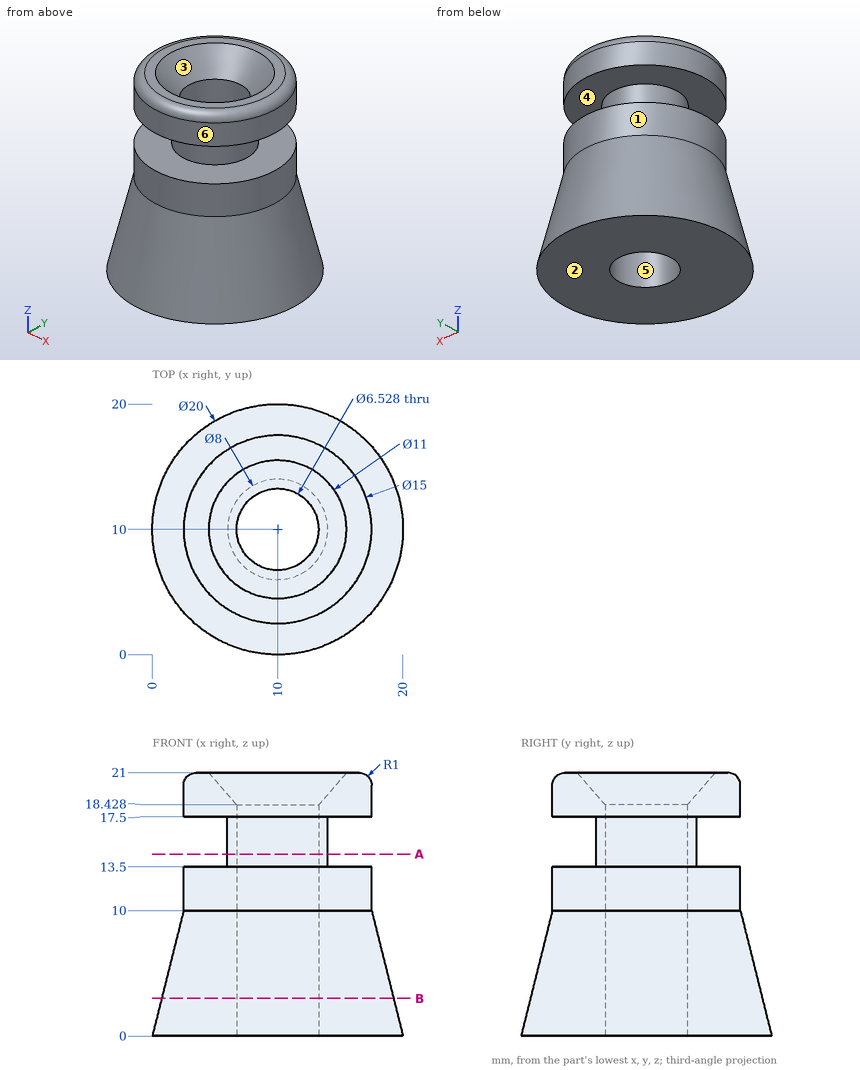
The drawing under review shows one solid part. Ordinate dimensions are in mm from its lowest x, y, z. A direction names the side the tool comes from. Round coordinates to 2 decimals unless told otherwise and drop trailing zeros. Write each loop counter-clockwise with the first axis right and the second up, starting at its lowest first coordinate (ties: lowest second). Pieces come first, ordered by that corner, then holes. Notation, with made-up numbers: (22.5, 60.5) -> (71.5, 60.5) arc R12 ccw to (71.5, 64.5) -> close; hole circle Ø4 at (-23, 38). An arc over 180 degrees is marked (long way). One line per question, with ' | ' between items. Start each with the question number.
(1) Tool access review of the marked faces 4, 5 and 6: name each direction out of +Z, -Z, +X, -X, +Y, -Y from which nothing blocks a thin tool from reaching the whole face with its end or side.
(2) Mouldability with a two-part tool opening along Y and no side actions: class the marked faces 1, 2 and 3 as released by +Y, released by -Y, zero draft, split by the parting line, or undercut.
(3) Insertion check: P1, Ø1.5, axis at y = 11, z = 5, coming from the -X side (1 decimal); P2, Ø12, axis at x = 12.5, z = 8.5, coming from the +Y side; P3, Ø2, axis at y = 12, z = 13, coming from the -X side. Each pin has a flat end and moves straight along its axis. Give the tip position at first contact, or say it passes through.
(4) Add section A-A, the plane z = 14.5. Write out the cut boundary in (x, y), plus the area to 3 significant figures.
(5) Add section B-B, the plane z = 3. Write out the cut boundary in (x, y).
(6) For line 1 along Y through (x, z) = (10, 11.75); line 2 along Z through (x, y) = (13, 4.5); line 3 along Y through (x, z) = (12.75, 1.5) (1 decimal), list the stretches that pass through material, from the lowest coordinate up. Write a range as from..to.
Answer list:
1) face 4: none | face 5: +Z, -Z | face 6: +Z
2) face 1: split by the parting line | face 2: zero draft | face 3: undercut
3) P1: x = 1.1 | P2: y = 19.28 | P3: x = 2.57
4) outline: circle Ø8 at (10, 10); hole circle Ø6.53 at (10, 10) | area: 16.8 mm²
5) outline: circle Ø18.5 at (10, 10); hole circle Ø6.53 at (10, 10)
6) line 1: 2.5..6.74, 13.26..17.5 | line 2: 0..13.5, 17.5..21 | line 3: 0.8..8.2, 11.8..19.2
